Model file for the job. Use its own axes, mm. Face numbers are marked on the shaded views. A direction names the side the tool comes from. Coordinates: 2 decimals unless noted, no trailing zeros. Loops run counter-clockwise (first coordinate to the right, second up) from the corner with the lowest first, then second, coordinate; pieces in that order, holes last.
Autodesk Inventor part; units mm, degrees
ref_plane "РабПлоскость1" through (0, 0, 0) normal (0, 0, 1) x (1, 0, 0)
ref_plane "РабПлоскость4" through (0, 0, 40) normal (0, 0, 1) x (1, 0, 0)
ref_plane "YZ Plane" through (0, 0, 0) normal (1, 0, 0) x (0, 1, 0)
sketch "Эскиз1" plane through (0, 0, 0) normal (0, 0, 1) x (1, 0, 0)
  line L0 (0, 0) -> (75, 0)
  line L1 (75, -50) -> (0, -50)
  line L2 (0, -50) -> (0, -45)
  arc A0 (75, -50) -> (75, 0) centre (75, -25) ccw
  line L3 (0, -25) -> (0, -15)
  line L4 (0, -15) -> (0, -35)
  line L5 (0, -35) -> (10, -35)
  line L6 (10, -45) -> (0, -45)
  line L7 (0, -15) -> (10, -15)
  line L8 (10, -5) -> (0, -5)
  arc A1 (10, -15) -> (10, -5) centre (10, -10) ccw
  arc A2 (10, -45) -> (10, -35) centre (10, -40) ccw
  line L9 (0, -5) -> (0, 0)
  line L10 (0, -35) -> (0, -15)
  circle A3 centre (50, -25) radius 12.5
  circle A4 centre (75, -25) radius 5
  line L11 (20, -25) -> (20, -21.5)
  line L12 (20, -21.5) -> (20, -28.5)
  line L13 (20, -28.5) -> (38, -28.5)
  line L14 (20, -21.5) -> (38, -21.5)
sketch "Эскиз2" plane through (0, 0, 0) normal (0, 1, 0) x (-1, 0, 0)
  point P0 (0, 0)
sketch "Эскиз3" plane through (0, 0, 0) normal (0, 1, 0) x (-1, 0, 0)
  line L0 (0, 0) -> (0, 10)
  line L1 (0, 10) -> (-20, 10)
  line L2 (-20, 10) -> (-37.5, 10)
  line L3 (-37.5, 10) -> (-37.5, 20)
  line L4 (-37.5, 20) -> (-20, 10)
  line L5 (-44.031, 23.732) -> (-37.5, 20)
  line L6 (-44.031, 23.732) -> (-44.031, 33.732)
  line L7 (-44.031, 33.732) -> (-20, 33.732)
  line L8 (-20, 33.732) -> (-20, 10)
  dimension "d24" = 10
  dimension "d25" = 20
  dimension "d26" = 17.5
  dimension "d27" = 10
  dimension "d28" = 10
sketch "Эскиз4" plane through (0, 0, 0) normal (0, 1, 0) x (-1, 0, 0)
  point P0 (0, 0)
ref_plane "РабПлоскость1" through (0, 0, 0) normal (0, 0, 1) x (1, 0, 0)
sketch "Эскиз5" plane through (0, 0, 0) normal (0, 0, 1) x (1, 0, 0)
  circle A0 centre (50, -25) radius 12.5
  point P0 (0, 0)
ref_plane "РабПлоскость2" through (0, 0, 0) normal (0, 0, 1) x (1, 0, 0)
sketch "Эскиз6" plane through (0, 0, 0) normal (0, 0, 1) x (1, 0, 0)
  line L0 (20, -21.5) -> (20, -28.5)
  line L1 (20, -28.5) -> (39.2288, -28.5)
  line L2 (39.2288, -28.5) -> (39.2288, -21.5)
  line L3 (39.2288, -21.5) -> (20, -21.5)
  point P0 (0, 0)
extrude "Выдавливание1" add sketch "Эскиз1" along normal blind 10
extrude "Выдавливание2" add sketch "Эскиз6" along normal blind 25
extrude "Выдавливание3" cut sketch "Эскиз3" against normal blind 35 contours L4 L5 L6 L7 L8
ref_plane "РабПлоскость3" through (0, 0, 0) normal (0, 0, 1) x (1, 0, 0)
sketch "Эскиз7" plane through (0, 0, 0) normal (0, 0, 1) x (1, 0, 0)
  circle A0 centre (50, -25) radius 12.5
  point P0 (0, 0)
extrude "Выдавливание4" cut sketch "Эскиз7" along normal blind 25
extrude "Выдавливание5" add sketch "Эскиз5" along normal blind 25
ref_plane "РабПлоскость4" through (0, 0, 40) normal (0, 0, 1) x (1, 0, 0)
sketch "Эскиз8" plane through (0, 0, 40) normal (0, 0, 1) x (1, 0, 0)
  circle A0 centre (50, -25) radius 8
  point P0 (0, 0)
extrude "Выдавливание6" cut sketch "Эскиз8" against normal blind 70
thread "Резьба1"
chamfer "Фаска1" distance 2 angle 45 1 edges at (42, -25, 25)
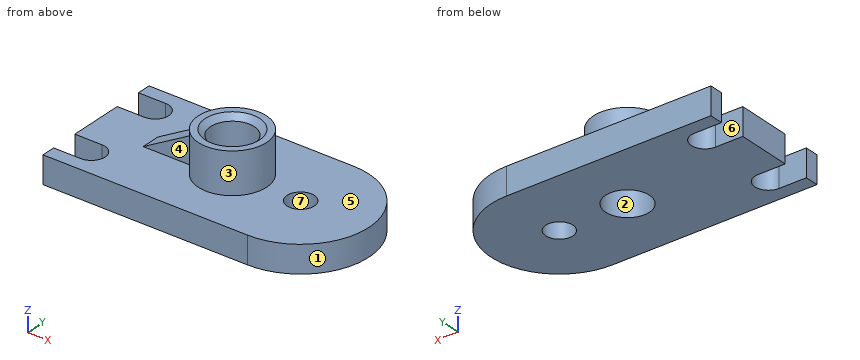
Q1. Slice it at B-B (x = 50). List the corners of the cut face in (y, z), and give its area (3 significant figures).
Answers:
outline: (-50, 0) - (-33, 0) - (-33, 23) - (-35, 25) - (-37.5, 25) - (-37.5, 10) - (-50, 10) - close; (-17, 0) - (0, 0) - (0, 10) - (-12.5, 10) - (-12.5, 25) - (-15, 25) - (-17, 23) - close
area: 471 mm2
Q2. Drill centre lines: line 1 (Y direction, x = 8, z = 3); line 2 (Y direction, x = 75, z = 5.5); line 3 (Y direction, x = 50, z = 7). Where is each one in solid material? Low to high.
Answers:
line 1: y = -50 to -45, -35 to -15, -5 to 0
line 2: y = -50 to -30, -20 to 0
line 3: y = -50 to -33, -17 to 0
Q3. Which spindle directions (+Z, -Z, +X, -X, +Y, -Y) get a long thin tool onto all of the face, cutting with end or side? Do the marked faces 4, 5, 6 and 7. Say none if no direction does.
Answers:
face 4: +Z, -X, -Y
face 5: +Z
face 6: +Z, -Z, -X
face 7: +Z, -Z
Q4. Mould opens along X. For the marked faces 1, 2 and 3 say: +X half, -X half, draft (parallel to the pull), parting line (faces both ways), or undercut.
Answers:
face 1: +X half
face 2: undercut
face 3: parting line
Q5. Slice it at C-C (z = 2.25). List the corners of the cut face in (x, y), and give its area (3 significant figures).
Answers:
outline: (0, -50) - (75, -50) arc R25 ccw to (75, 0) - (0, 0) - (0, -5) - (10, -5) arc R5 cw to (10, -15) - (0, -15) - (0, -35) - (10, -35) arc R5 cw to (10, -45) - (0, -45) - close; hole circle Ø16 at (50, -25); hole circle Ø10 at (75, -25)
area: 4,170 mm2
Q6. Flat gauge pins, fed straight in: P1, Ø3, axis at x = 38, z = 13.5, coming from the -Y side; P2, Ø1, axis at x = 75, y = -21, coming from the +Z side; P3, Ø8, axis at x = 28, z = 17, coming from the -Y side; P4, Ø16, axis at x = 75, y = -25, coming from the +Z side. Where does each tip first touch, or does it go through?
Answers:
P1: stops at y = -31.78
P2: passes through
P3: stops at y = -28.5
P4: stops at z = 10
Q7. Slice it at A-A (y = -25). List the corners of the cut face in (x, z).
Answers:
outline: (0, 0) - (42, 0) - (42, 23) - (40, 25) - (37.5, 25) - (37.5, 20) - (20, 10) - (0, 10) - close; (58, 0) - (70, 0) - (70, 10) - (62.5, 10) - (62.5, 25) - (60, 25) - (58, 23) - close; (80, 0) - (100, 0) - (100, 10) - (80, 10) - close
Q8. Slice it at D-D (z = 15). List the corners of the cut face in (x, y), and give its area (3 significant figures).
Answers:
outline: (28.75, -28.5) - (38, -28.5) arc R12.5 ccw (long way) to (38, -21.5) - (28.75, -21.5) - close; hole circle Ø16 at (50, -25)
area: 352 mm2
